Build history of the part. All positions in model axes, mm. A direction names the side the tool comes from. Coordinates: 2 decimals unless noted, no trailing zeros. Loops run counter-clockwise (first coordinate to the right, second up) from the corner with the lowest first, then second, coordinate; pieces in that order, holes last. Notation, with made-up numbers: (84.25, -27.5) - (120.25, -27.5) arc R22 cw to (120.25, -15.5) - close; hole circle Ø11 at (71.25, 59.5). An arc over 180 degrees is marked (long way). One line per item, written item: value.
```python
from build123d import *

# Parameters (mm, degrees)
SKETCH1_R           = 20.3
SKETCH1_R_2         = 17
BOSS_EXTRUDE1_DEPTH = 2
SKETCH2_R           = 19.8
SKETCH2_R_2         = 18.88
BOSS_EXTRUDE2_DEPTH = 4
CHAMFER2_SIZE       = 0.4
CUT_EXTRUDE1_START  = -0.5
SKETCH3_R           = 18.88
CUT_EXTRUDE1_DEPTH  = 0.5
FILLET1_R           = 1


with BuildPart() as part:
    # Sketch1 → Boss-Extrude1 (new body)
    with BuildSketch(Plane.XY):
        Circle(SKETCH1_R)
        Circle(SKETCH1_R_2, mode=Mode.SUBTRACT)
    extrude(amount=-BOSS_EXTRUDE1_DEPTH)

    # Sketch2 → Boss-Extrude2 (add)
    with BuildSketch(Plane(origin=(0, 0, -2), x_dir=(-1, 0, 0), z_dir=(0, 0, -1))):
        with Locations(Location((0, 0, 0), (0, 0, 180))):
            Circle(SKETCH2_R)
        Circle(SKETCH2_R_2, mode=Mode.SUBTRACT)
    extrude(amount=BOSS_EXTRUDE2_DEPTH)

    # Chamfer2
    chamfer2_edges = [part.edges().sort_by_distance(p)[0] for p in [
        (-17, 0, 0),
    ]]
    chamfer(chamfer2_edges, length=CHAMFER2_SIZE)

    # Sketch3 → Cut-Extrude1 (cut)
    with BuildSketch(Plane(origin=(0, 0, -2), x_dir=(-1, 0, 0), z_dir=(0, 0, -1)).offset(CUT_EXTRUDE1_START)):
        Circle(SKETCH3_R)
    extrude(amount=CUT_EXTRUDE1_DEPTH, mode=Mode.SUBTRACT)

    # Fillet1
    fillet1_edges = [part.edges().sort_by_distance(p)[0] for p in [
        (-20.3, 0, 0),
    ]]
    fillet(fillet1_edges, radius=FILLET1_R)


solid = part.part
```
Item 1: Pull direction Y, two halves, no side cores. Call faces 3 (the face through (17, 3, -1.5)), 4 (the face through (-10.1, 14.4, 0)), 5 (the face through (9.139, 14.334, -0.942)), 6 (the face through (-16.11, -12.35, -1.49)): released by +Y, released by -Y, zero draft, split by the parting line, or undercut.
Check result:
face 3: undercut
face 4: zero draft
face 5: undercut
face 6: split by the parting line
Item 2: Cut at A-A, the plane y = 0. Write the cut outline in (x, z).
Check result:
outline: (-20.3, -2) - (-19.8, -2) - (-19.8, -6) - (-18.88, -6) - (-18.88, -1.5) - (-17, -1.5) - (-17, -0.4) - (-17.4, 0) - (-19.3, 0) arc R1 ccw to (-20.3, -1) - close; (17, -1.5) - (18.88, -1.5) - (18.88, -6) - (19.8, -6) - (19.8, -2) - (20.3, -2) - (20.3, -1) arc R1 ccw to (19.3, 0) - (17.4, 0) - (17, -0.4) - close
Item 3: Probe probe 1 along Y at (x, z) = (0, -1.3); probe 2 along Y at (x, z) = (0, -4.55); probe 3 along Z at (x, y) = (-13.5, -12). List the from-to ranges inside material, lowest first. Write a range as from..to.
Check result:
probe 1: y = -20.3..-17, 17..20.3
probe 2: y = -19.8..-18.88, 18.88..19.8
probe 3: z = -1.5..0
Item 4: Drop flat-ended pins along their axis: P1, Ø20.5, axis at x = 0, y = 0, coming from the -Z side; P2, Ø10, axis at x = 10, y = 7, coming from the -Z side. Give the stop position or say it passes through.
Check result:
P1: passes through
P2: stops at z = -1.5
Item 5: Cut at C-C, the plane z = -4.6. Write the cut outline in (x, y).
Check result:
outline: circle Ø39.6 at (0, 0); hole circle Ø37.76 at (0, 0)
Item 6: Tool access for faces 1 (the face through (18.9, -5.9, -4)), 2 (the face through (18, 7, -6)): list every direction of +Z, -Z, +X, -X, +Y, -Y with a clear straight run to the whole face (end or side of a thin tool).
Check result:
face 1: -Z
face 2: -Z, +X, -X, +Y, -Y
